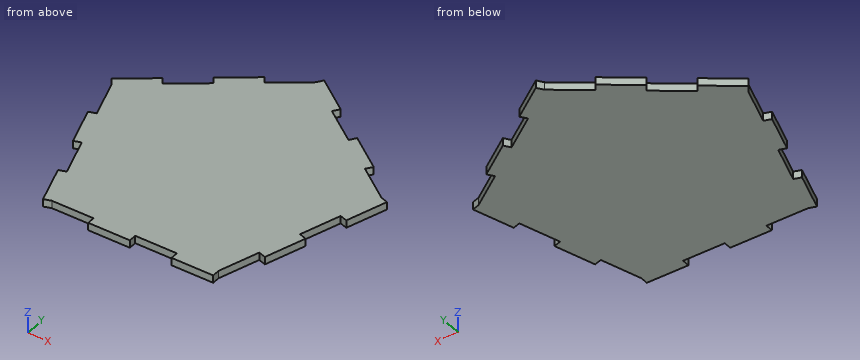
from build123d import *

# Parameters (mm, degrees)
F2_DEPTH = 3
F4_DEPTH = 3


with BuildPart() as f2:
    # F0 (on Top) → F2 (new body)
    with BuildSketch(Plane.XY):
        Polygon((53.4142809913, 17.3553519542), (0, 56.1630986972), (-53.4142809913, 17.3553519542), (-33.0118411373, -45.4369013028), (33.0118411373, -45.4369013028), align=None)
    extrude(amount=F2_DEPTH)

    # F3 (on face) → F4 (join)
    with BuildSketch(Plane.XY.offset(3)):
        Polygon((15.1169260047, 48.8882129946), (1.7633557569, 58.5901496803), (0, 56.1630986972), (-13.3535702478, 46.4611620115), (-15.1169260047, 48.8882129946), (-28.4704962525, 39.1862763088), (-26.7071404957, 36.7592253257), (-40.0607107435, 27.0572886399), (-41.8240665004, 29.4843396231), (-55.1776367482, 19.7824029373), (-53.4142809913, 17.3553519542), (-48.3136710278, 1.6572886399), (-51.1668405767, 0.7302376568), (-46.0662306132, -14.9678256574), (-43.2130610643, -14.0407746743), (-38.1124511008, -29.7388379885), (-40.9656206497, -30.6658889717), (-35.8650106861, -46.3639522859), (-33.0118411373, -45.4369013028), (-16.5059205686, -45.4369013028), (-16.5059205686, -48.4369013028), (0, -48.4369013028), (0, -45.4369013028), (16.5059205686, -45.4369013028), (16.5059205686, -48.4369013028), (33.0118411373, -48.4369013028), (33.0118411373, -45.4369013028), (38.1124511008, -29.7388379885), (40.9656206497, -30.6658889717), (46.0662306132, -14.9678256574), (43.2130610643, -14.0407746743), (48.3136710278, 1.6572886399), (51.1668405767, 0.7302376568), (56.2674505402, 16.4283009711), (53.4142809913, 17.3553519542), (40.0607107435, 27.0572886399), (41.8240665004, 29.4843396231), (28.4704962525, 39.1862763088), (26.7071404957, 36.7592253257), (13.3535702478, 46.4611620115), align=None)
    extrude(amount=-F4_DEPTH)


solid = f2.part
Design review of the part built by this model. Coordinates are the model's own, in mm. Round coordinates to 2 decimals unless told otherwise and drop trailing zeros. Loops run counter-clockwise (first coordinate to the right, second up) from the corner with the lowest first, then second, coordinate; pieces in that order, holes last. Notation, with made-up numbers: M 67,42 L 71,42 A18 ccw 71,65 Z; hole C -16,25.5 d10. An arc over 180 degrees is marked long. Answer as a JSON object with one key per item and string values.
Item 1: We need section B-B on y = 4.5. Give the boundary of the cut face in (x, z), and give its area (3 significant figures).
Answer sheet:
{"outline": "M -49.24,0 L 52.39,0 L 52.39,3 L -49.24,3 Z", "area": "305 mm^2"}
Item 2: Wall thickness on L1, parallel to X at y = 48, z = 1.45; L2, parallel to X at y = 39, z = 1.05; L3, parallel to Y at x = -19, z = 1.05: over which ranges is each line inside the solid? List them lowest first. Write a range as from..to.
Answer sheet:
{"L1": "x = -16.34..-14.47, -11.24..14.47", "L2": "x = -28.34..23.62, 28.34..28.73", "L3": "y = -45.44..46.07"}
Item 3: We need section A-A on x = 20.5. Give the boundary of the cut face in (y, z).
Answer sheet:
{"outline": "M -48.44,0 L 41.27,0 L 41.27,3 L -48.44,3 Z"}
Item 4: Clearance check with flat-ended pins moving along their axes: P1, Ø1.5, axis at y = -2.5, z = 0.5, coming from the +X side; P2, Ø0.9, axis at y = -47, z = 1.5, coming from the -X side; P3, Ø0.9, axis at y = -47.5, z = 1, coming from the +X side. State where each tip first meets the part, or that it passes through.
Answer sheet:
{"P1": "stops at x = 47.21", "P2": "stops at x = -16.51", "P3": "stops at x = 33.01"}
